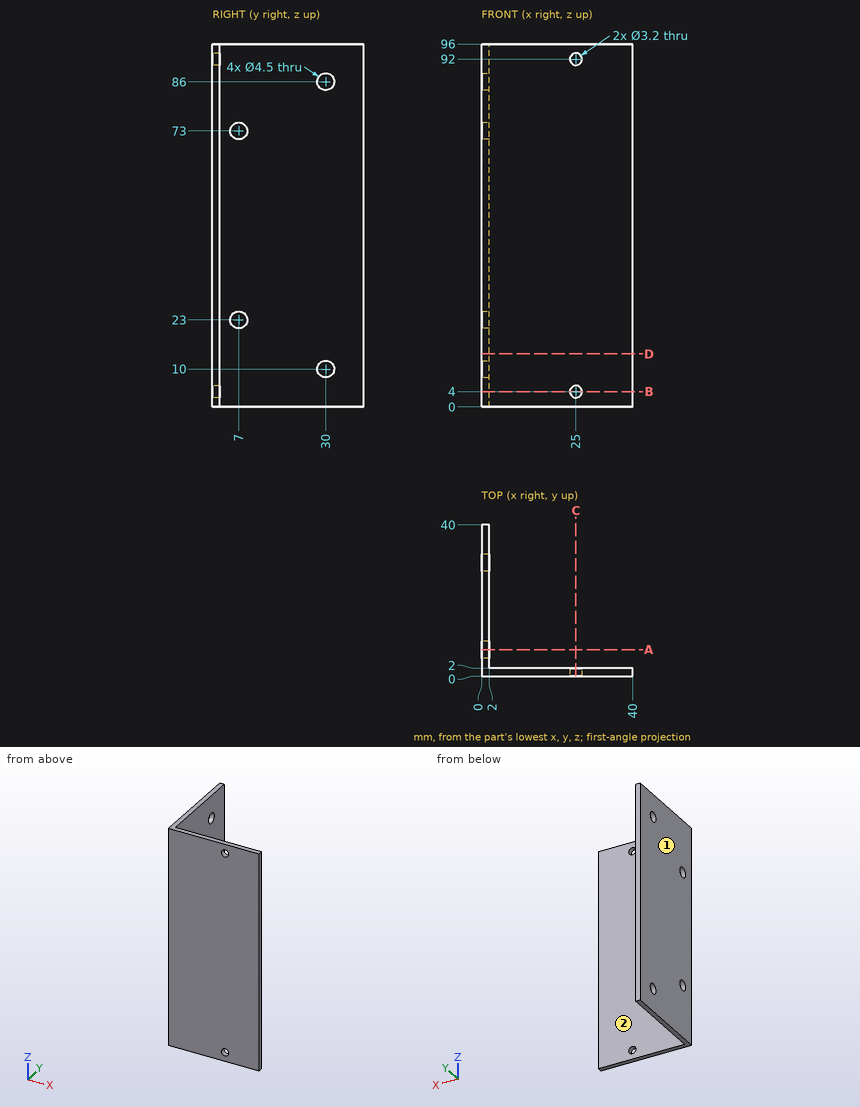
Input: dimensioned drawing with shaded views. Units: mm. Origin: part minimum x, y, z. A direction names the side the tool comes from. Round coordinates to 2 decimals unless told otherwise and drop trailing zeros. Order: outer loops, then holes, each group sorted by start corner. A loop starts at its lowest first (then second) coordinate and runs counter-clockwise, first axis right, second up. Notation, with made-up numbers: (36, 66.25) - (72, 66.25) arc R32 cw to (72, 104.25) - close; hole circle Ø6 at (-31.75, -1.5). An arc over 180 degrees is marked (long way). Write item = value, one per line. Start each with the question number.
Q1. Access query for the marked faces 1 and 2. Directions: +Z, -Z, +X, -X, +Y, -Y. A direction counts if a zero-diameter tool reaches every point of the face in a straight line with its end or side. Return the directions, or none.
Q2. Pin query (flat end, axial travel): pin 1 (4 mm diameter, centred on y = 30, z = 10, fed in from +X); pin 2 (1.5 mm diameter, centred on x = 11, z = 74.5, fed in from +Y); pin 3 (6 mm diameter, centred on y = 7, z = 55, fed in from +X). Return the tip coordinate at first contact, or that it passes through.
Q3. Cut plane A-A on y = 7. Return the cut outline in (x, z), and give its area (3 significant figures).
Q4. Cut plane B-B on z = 4. Return the cut outline in (x, y).
Q5. Cut plane C-C on x = 25. Return the cut outline in (y, z).
Q6. Cut plane D-D on z = 14. Return the cut outline in (x, y).
Q7. Ray query, line 1 (X direction, y = 0.8, z = 92); line 2 (Y direction, x = 1, z = 10); line 3 (X direction, y = 15, z = 78). Return the intervals inside material, ascending. Write a range as from..to.
Outcome:
q1.face_1 = +Z, -Z, -X, +Y, -Y
q1.face_2 = +Z, -Z, +X, +Y
q2.pin_1 = through
q2.pin_2 = 2
q2.pin_3 = 2
q3.outline = (0, 0) - (2, 0) - (2, 20.75) - (0, 20.75) - close; (0, 25.25) - (2, 25.25) - (2, 70.75) - (0, 70.75) - close; (0, 75.25) - (2, 75.25) - (2, 96) - (0, 96) - close
q3.area = 174 mm^2
q4.outline = (0, 0) - (23.4, 0) - (23.4, 2) - (2, 2) - (2, 40) - (0, 40) - close; (26.6, 0) - (40, 0) - (40, 2) - (26.6, 2) - close
q5.outline = (0, 0) - (2, 0) - (2, 2.4) - (0, 2.4) - close; (0, 5.6) - (2, 5.6) - (2, 90.4) - (0, 90.4) - close; (0, 93.6) - (2, 93.6) - (2, 96) - (0, 96) - close
q6.outline = (0, 0) - (40, 0) - (40, 2) - (2, 2) - (2, 40) - (0, 40) - close
q7.line_1 = 0..23.4, 26.6..40
q7.line_2 = 0..27.75, 32.25..40
q7.line_3 = 0..2
